Input: dimensioned drawing with shaded views. Units: mm. Origin: part minimum x, y, z. Coordinates: 2 decimals unless noted, no trailing zeros. Write each loop counter-clockwise with the first axis right and the second up, starting at its lowest first coordinate (ties: lowest second). Pieces come first, ordered by that corner, then holes. Notation, with made-up numbers: M 61,15.5 L 70,15.5 A16 ccw 70,45.5 Z; hole C -25.75,64 d10. An arc over 180 degrees is marked long. Use one line per item in the form item = value.
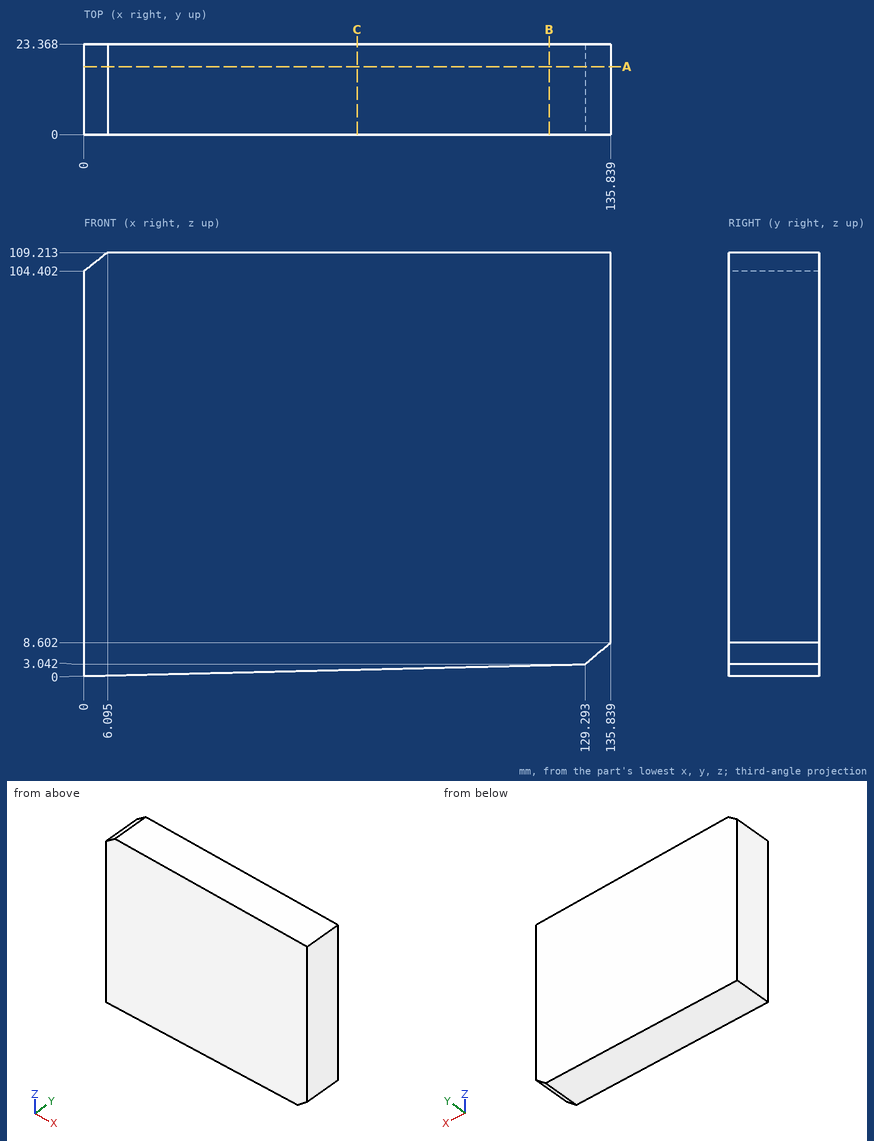
(1) Section query C-C on x = 70.5. Return the cut outline in (y, z).
Computed:
outline = M 0,1.66 L 23.37,1.66 L 23.37,109.21 L 0,109.21 Z
(2) Section query A-A on y = 17.5. Return the cut outline in (x, z) (1 decimal).
Computed:
outline = M 0,0 L 129.3,3 L 135.8,8.6 L 135.8,109.2 L 6.1,109.2 L 0,104.4 Z
(3) Section query B-B on x = 120. Return the cut outline in (y, z), plus the area to 3 significant figures.
Computed:
outline = M 0,2.82 L 23.37,2.82 L 23.37,109.21 L 0,109.21 Z
area = 2,490 mm^2
(4) Line query: probe 1 along Z at (x, y) = (13, 6) (1 decimal); probe 2 along Z at (x, y) = (115, 19) (1 decimal); probe 3 along X at (y, z) = (3, 5.5) (1 decimal). Output: solid intervals per line, ascending.
Computed:
probe_1 = 0.3 to 109.2
probe_2 = 2.7 to 109.2
probe_3 = 0 to 132.2
